Input: part model. Units: mm. Frame: model coordinates. Round coordinates to 2 decimals unless told otherwise and drop trailing zeros. Write each loop counter-clockwise with the first axis right and the second up, starting at its lowest first coordinate (ties: lowest second). Pieces come first, ordered by that corner, then holes. Notation, with made-up numbers: (88, 46.25) - (131, 46.25) arc R12 ccw to (131, 65.25) - close; hole circle Ø8 at (55, 11). An arc over 180 degrees is marked (long way). Use one line per item in the form item = value.
```python
from build123d import *

# Parameters (mm, degrees)
SKETCH2_R               = 15
BOSS_EXTRUDE1_DEPTH     = 10
SKETCH3_R               = 10
CUT_EXTRUDE1_DEPTH      = 24.452078799
CUT_EXTRUDE2_DEPTH      = 24.452078799
CUT_EXTRUDE2_DEPTH_BACK = 24.452078799
SKETCH4_R               = 2.5


with BuildPart() as part:
    # Sketch2 → Boss-Extrude1 (new body)
    with BuildSketch(Plane(origin=(0, 0, 0), x_dir=(1, 0, 0), z_dir=(0, 1, 0))):
        with Locations(Location((0, 0, 0), (0, 0, 270))):
            Circle(SKETCH2_R)
    extrude(amount=BOSS_EXTRUDE1_DEPTH)

    # Sketch3 → Cut-Extrude1 (cut, through all)
    with BuildSketch(Plane(origin=(0, 10, 0), x_dir=(1, 0, 0), z_dir=(0, 1, 0))):
        with Locations(Location((0, 0, 0), (0, 0, 270))):
            Circle(SKETCH3_R)
    extrude(amount=-CUT_EXTRUDE1_DEPTH, mode=Mode.SUBTRACT)

    # Sketch4 → Cut-Extrude2 (cut, two sides: drawn at the far end of the back side and taken through both)
    with BuildSketch(Plane.XY.offset(-CUT_EXTRUDE2_DEPTH_BACK)):
        with Locations((0, 5)):
            Circle(SKETCH4_R)
    extrude(amount=CUT_EXTRUDE2_DEPTH + CUT_EXTRUDE2_DEPTH_BACK, mode=Mode.SUBTRACT)


solid = part.part
```
(1) First-contact query: pin 1 Ø1.5 at (y, z) = (1.5, -4) entering from -X; pin 2 Ø4 at (y, z) = (7, -10.5) entering from +X; pin 3 Ø1 at (x, y) = (5, 7) entering from -Z. Flat tips, straight axial feed; report the tip coordinate or a pass-through.
Derived:
pin_1 = -14.64
pin_2 = 12.36
pin_3 = -14.31
(2) Cut plane A-A on x = 0. Output: boundary loops of the cut face in (y, z), then the cut area to 3 significant figures.
Derived:
outline = (0, -15) - (2.5, -15) - (2.5, -10) - (0, -10) - close; (0, 10) - (2.5, 10) - (2.5, 15) - (0, 15) - close; (7.5, -15) - (10, -15) - (10, -10) - (7.5, -10) - close; (7.5, 10) - (10, 10) - (10, 15) - (7.5, 15) - close
area = 50.0 mm^2
(3) Cut plane D-D on z = 12. Output: boundary loops of the cut face in (x, y).
Derived:
outline = (-9, 0) - (9, 0) - (9, 10) - (-9, 10) - close; hole circle Ø5 at (0, 5)
(4) Cut plane B-B on z = 0. Output: boundary loops of the cut face in (x, y), then the cut area to 3 significant figures.
Derived:
outline = (-15, 0) - (-10, 0) - (-10, 10) - (-15, 10) - close; (10, 0) - (15, 0) - (15, 10) - (10, 10) - close
area = 100 mm^2
(5) Cut plane C-C on y = 6. Output: boundary loops of the cut face in (x, z).
Derived:
outline = (-2.29, -14.82) - (-2.29, -9.73) arc R10 cw to (-2.29, 9.73) - (-2.29, 14.82) arc R15 ccw to start; (2.29, -14.82) arc R15 ccw to (2.29, 14.82) - (2.29, 9.73) arc R10 cw to (2.29, -9.73) - close
(6) Material intervals for L1, parallel to Y at x = 0, z = 10.9; L2, parallel to X at y = 5.75, z = -10; L3, parallel to Y at x = -2, z = 10.5, sorted ascending.
Derived:
L1 = 0 to 2.5, 7.5 to 10
L2 = -11.18 to -2.38, 2.38 to 11.18
L3 = 0 to 3.5, 6.5 to 10
(7) Draft query along Y for faces 1 (the face through (-10, 10, 3)), 2 (the face through (-10, 0, 3)), 3 (the face through (2.385, 5.751, 12.304)). Return one class per face: released by +Y, released by -Y, zero draft, split by the parting line, or undercut.
Derived:
face_1 = released by +Y
face_2 = released by -Y
face_3 = undercut
